```python
from build123d import *

# Parameters (mm, degrees)
BOSS_EXTRUDE1_DEPTH = 1.27
SKETCH2_R           = 10.16
SKETCH2_R_2         = 1.5875
CUT_EXTRUDE1_DEPTH  = 50.5872797


with BuildPart() as part:
    # Sketch1 → Boss-Extrude1 (new body)
    with BuildSketch(Plane(origin=(0, 0, 0), x_dir=(1, 0, 0), z_dir=(0, 1, 0))):
        with BuildLine():
            Line((29.972, -35.052), (-29.972, -35.052))
            ThreePointArc((-29.972, -35.052), (-33.564102448, -33.564102448), (-35.052, -29.972))
            Line((-35.052, -29.972), (-35.052, 29.972))
            ThreePointArc((-35.052, 29.972), (-33.564102448, 33.564102448), (-29.972, 35.052))
            Line((-29.972, 35.052), (29.972, 35.052))
            ThreePointArc((29.972, 35.052), (33.564102448, 33.564102448), (35.052, 29.972))
            Line((35.052, 29.972), (35.052, -29.972))
            ThreePointArc((35.052, -29.972), (33.564102448, -33.564102448), (29.972, -35.052))
        make_face()
    extrude(amount=BOSS_EXTRUDE1_DEPTH)

    # Sketch2 → Cut-Extrude1 (cut, through all)
    with BuildSketch(Plane(origin=(0, 1.27, 0), x_dir=(1, 0, 0), z_dir=(0, 1, 0))):
        with Locations(Location((0, 0, 0), (0, 0, 270))):
            Circle(SKETCH2_R)
        with Locations(Location((20.833792189, 0, 0), (0, 0, 270))):
            Circle(SKETCH2_R_2)
        with Locations(Location((30.988, 0, 0), (0, 0, 270))):
            Circle(SKETCH2_R_2)
        with Locations(Location((-20.833792189, 0, 0), (0, 0, 90))):
            Circle(SKETCH2_R_2)
        with Locations(Location((-30.988, 0, 0), (0, 0, 90))):
            Circle(SKETCH2_R_2)
        with Locations(Location((0, -20.828, 0), (0, 0, 270))):
            Circle(SKETCH2_R_2)
        with Locations(Location((0, 30.988, 0), (0, 0, 90))):
            Circle(SKETCH2_R_2)
        with Locations(Location((0, 20.828, 0), (0, 0, 90))):
            Circle(SKETCH2_R_2)
        with Locations(Location((-15.266435406, -15.266435406, 0), (0, 0, 270))):
            Circle(SKETCH2_R_2)
        with Locations(Location((-22.450640303, -22.450640303, 0), (0, 0, 270))):
            Circle(SKETCH2_R_2)
        with Locations(Location((-28.800640303, -22.450640303, 0), (0, 0, 270))):
            Circle(SKETCH2_R_2)
        with Locations(Location((-22.450640303, -28.800640303, 0), (0, 0, 270))):
            Circle(SKETCH2_R_2)
        with Locations(Location((28.800640303, -22.450640303, 0), (0, 0, 90))):
            Circle(SKETCH2_R_2)
        with Locations(Location((22.450640303, -28.800640303, 0), (0, 0, 90))):
            Circle(SKETCH2_R_2)
        with Locations(Location((22.450640303, -22.450640303, 0), (0, 0, 90))):
            Circle(SKETCH2_R_2)
        with Locations(Location((15.266435406, -15.266435406, 0), (0, 0, 90))):
            Circle(SKETCH2_R_2)
        with Locations(Location((28.800640303, 22.450640303, 0), (0, 0, 270))):
            Circle(SKETCH2_R_2)
        with Locations(Location((22.450640303, 28.800640303, 0), (0, 0, 270))):
            Circle(SKETCH2_R_2)
        with Locations(Location((22.450640303, 22.450640303, 0), (0, 0, 270))):
            Circle(SKETCH2_R_2)
        with Locations(Location((15.266435406, 15.266435406, 0), (0, 0, 270))):
            Circle(SKETCH2_R_2)
        with Locations(Location((-22.450640303, 28.800640303, 0), (0, 0, 90))):
            Circle(SKETCH2_R_2)
        with Locations(Location((-28.800640303, 22.450640303, 0), (0, 0, 90))):
            Circle(SKETCH2_R_2)
        with Locations(Location((-15.266435406, 15.266435406, 0), (0, 0, 90))):
            Circle(SKETCH2_R_2)
        with Locations(Location((-22.450640303, 22.450640303, 0), (0, 0, 90))):
            Circle(SKETCH2_R_2)
        with Locations(Location((0, -30.988, 0), (0, 0, 270))):
            Circle(SKETCH2_R_2)
    extrude(amount=-CUT_EXTRUDE1_DEPTH, mode=Mode.SUBTRACT)


solid = part.part
```
The listing builds one solid part. Answer for the finished solid, in the listing's coordinates (mm). Coordinates: 2 decimals unless noted, no trailing zeros. Write each loop counter-clockwise with the first axis right and the second up, starting at its lowest first coordinate (ties: lowest second). Pieces come first, ordered by that corner, then holes. Notation, with made-up numbers: (39, 64) - (53, 64) arc R18 ccw to (53, 68) - close; hole circle Ø1 at (85, 31.25). An arc over 180 degrees is marked (long way). Return JSON: item names as keys, results as strings. Group by question number.
Q1. The part is cut by section B-B on x = 0. Write down the section's boundary in (y, z).
Q2. The part is cut by section A-A on z = 0. Write down the section's boundary in (x, y).
Q3. Flat-ended cylindrical pins translate along their axes: pin 1 Ø4 at (x, z) = (0, 20.828) entering from -Y; pin 2 Ø1.9 at (x, z) = (-22.45, -22.45) entering from -Y. Find the tip coordinate at first contact, or state that the pin passes through.
Q4. The part is cut by section C-C on y = 0.75. State how many separate pieces and enclosed holes the cut face has, and give its area (3 significant figures).
Q5. Find the intervals of material crossed by line 1 along Z through (x, y) = (14, 1.1); line 2 along X through (y, z) = (0.55, -21); line 3 along Z through (x, y) = (-28.5, 0.1), in increasing order. Write a range as [from, to].
Q6. For a pull along X with two mould halves and no side action, classify faces 1 (the cylindrical face through (-0.07, 0.644, -29.402)), 2 (the flat face through (8, 1.27, -8)), 3 (the cylindrical face through (-33.603, 0.626, -33.524)) as +X half, -X half, draft (parallel to the pull), parting line (faces both ways), or undercut.
Evaluation:
{
 "1": {"outline": "(0, -35.05) - (1.27, -35.05) - (1.27, -32.58) - (0, -32.58) - close; (0, -29.4) - (1.27, -29.4) - (1.27, -22.42) - (0, -22.42) - close; (0, -19.24) - (1.27, -19.24) - (1.27, -10.16) - (0, -10.16) - close; (0, 10.16) - (1.27, 10.16) - (1.27, 19.24) - (0, 19.24) - close; (0, 22.42) - (1.27, 22.42) - (1.27, 29.4) - (0, 29.4) - close; (0, 32.58) - (1.27, 32.58) - (1.27, 35.05) - (0, 35.05) - close"},
 "2": {"outline": "(-35.05, 0) - (-32.58, 0) - (-32.58, 1.27) - (-35.05, 1.27) - close; (-29.4, 0) - (-22.42, 0) - (-22.42, 1.27) - (-29.4, 1.27) - close; (-19.25, 0) - (-10.16, 0) - (-10.16, 1.27) - (-19.25, 1.27) - close; (10.16, 0) - (19.25, 0) - (19.25, 1.27) - (10.16, 1.27) - close; (22.42, 0) - (29.4, 0) - (29.4, 1.27) - (22.42, 1.27) - close; (32.58, 0) - (35.05, 0) - (35.05, 1.27) - (32.58, 1.27) - close"},
 "3": {"pin 1": "stops at y = 0", "pin 2": "passes through"},
 "4": {"separate pieces": "1", "enclosed holes": "25", "area": "4,380 mm2"},
 "5": {"line 1": "z = [-35.05, -16.22], [-14.31, 14.31], [16.22, 35.05]", "line 2": "x = [-35.05, -29.45], [-28.16, -23.1], [-21.81, -1.58], [1.58, 21.81], [23.1, 28.16], [29.45, 35.05]", "line 3": "z = [-35.05, -24.01], [-20.89, 20.89], [24.01, 35.05]"},
 "6": {"face 1": "undercut", "face 2": "draft", "face 3": "-X half"}
}
